```python
from build123d import *

# Parameters (mm, degrees)
F0_R     = 44.45
F1_DEPTH = 9.525
F2_R     = 2.0828
F3_DEPTH = 25.4
F4_R     = 3.6322
F5_DEPTH = 4.1656
F6_R     = 2.38125
F7_R     = 12.7


with BuildPart() as f1:
    # F0 (on Top) → F1 (new body)
    with BuildSketch(Plane.XY):
        with BuildLine():
            Line((-25.4, 90.4875), (-25.4, 43.994091))
            ThreePointArc((-25.4, 43.994091), (0, -50.8), (25.4, 43.994091))
            Line((25.4, 43.994091), (25.4, 90.4875))
            Line((25.4, 90.4875), (-25.4, 90.4875))
        make_face()
        Circle(F0_R, mode=Mode.SUBTRACT)
    extrude(amount=F1_DEPTH)

    # F2 (on face) → F3 (cut)
    with BuildSketch(Plane.XY.offset(9.525)):
        with Locations((-20.6375, 84.1375)):
            Circle(F2_R)
        with Locations((20.6375, 84.1375)):
            Circle(F2_R)
        with Locations((20.6375, 53.9623)):
            Circle(F2_R)
        with Locations((-20.6375, 53.9623)):
            Circle(F2_R)
    extrude(amount=-F3_DEPTH, mode=Mode.SUBTRACT)

    # F4 (on face) → F5 (cut)
    with BuildSketch(Plane.XY.offset(9.525)):
        with Locations((-20.6375, 84.1375)):
            Circle(F4_R)
        with Locations((20.6375, 84.1375)):
            Circle(F4_R)
        with Locations((20.6375, 53.9623)):
            Circle(F4_R)
        with Locations((-20.6375, 53.9623)):
            Circle(F4_R)
    extrude(amount=-F5_DEPTH, mode=Mode.SUBTRACT)

    # F6
    f6_edges = [f1.edges().sort_by_distance(p)[0] for p in [
        (-25.4, 90.4875, 4.7625),
        (25.4, 90.4875, 4.7625),
    ]]
    fillet(f6_edges, radius=F6_R)

    # F7
    f7_edges = [f1.edges().sort_by_distance(p)[0] for p in [
        (-25.4, 43.994091, 4.7625),
        (25.4, 43.994091, 4.7625),
    ]]
    fillet(f7_edges, radius=F7_R)


solid = f1.part
```
Design review of the part built by this model. Coordinates are the model's own, in mm. A direction names the side the tool comes from. Coordinates: 2 decimals unless noted, no trailing zeros. Loops run counter-clockwise (first coordinate to the right, second up) from the corner with the lowest first, then second, coordinate; pieces in that order, holes last.
Q1. We need section C-C on z = 1.5. State the section outline as (x, y) points, and give its area (3 significant figures).
Reported:
outline: (-30.48, 40.64) arc R50.8 ccw (long way) to (30.48, 40.64) arc R12.7 cw to (25.4, 50.8) - (25.4, 88.11) arc R2.38 ccw to (23.02, 90.49) - (-23.02, 90.49) arc R2.38 ccw to (-25.4, 88.11) - (-25.4, 50.8) arc R12.7 cw to start; hole circle Ø88.9 at (0, 0); hole circle Ø4.17 at (-20.64, 53.96); hole circle Ø4.17 at (-20.64, 84.14); hole circle Ø4.17 at (20.64, 53.96); hole circle Ø4.17 at (20.64, 84.14)
area: 3,980 mm2
Q2. Tool access review of faces 4 (the face through (25.4, 69, 5)), 5 (the face through (19.85, 50.416, 7.471)), 6 (the face through (-21.09, 51.93, 2.72)), 7 (the face through (-25.4, 70, 5)), 8 (the face through (0, 46, 9.525)): name each direction out of +Z, -Z, +X, -X, +Y, -Y from which nothing blocks a thin tool from reaching the whole face with its end or side.
Reported:
face 4: +Z, -Z, +X, +Y
face 5: +Z
face 6: +Z, -Z
face 7: +Z, -Z, -X, +Y
face 8: +Z, +X, -X, +Y, -Y
Q3. For pin 1 (4 mm diameter, centred on y = -14.5, z = 4, fed in from -X); pin 2 (3.5 mm diameter, centred on x = 20.64, y = 53.96, fed in from +Z); pin 3 (6.5 mm diameter, centred on x = 20.64, y = 84.14, fed in from +Z); pin 4 (2 mm diameter, centred on x = 14, z = 8, fed in from -Y), all flat-tipped, find the tip position at first contact; note any pin that passes through.
Reported:
pin 1: stops at x = -49.24
pin 2: passes through
pin 3: stops at z = 5.36
pin 4: stops at y = -49.11
Q4. To check wall thickness, follow line 1 (X direction, y = 51, z = 7.25); line 2 (Y direction, x = 20.5, z = 1.75); line 3 (X direction, y = 61, z = 3.5). State the ranges of each line that lie inside material, in increasing order.
Reported:
line 1: x = -25.4 to -22.74, -18.54 to 18.54, 22.74 to 25.4
line 2: y = -46.48 to -39.44, 39.44 to 51.88, 56.04 to 82.06, 86.22 to 90.49
line 3: x = -25.4 to 25.4
Q5. We need section B-B on y = 0. State the section outline as (x, z) points (3 decimals).
Reported:
outline: (-50.8, 0) - (-44.45, 0) - (-44.45, 9.525) - (-50.8, 9.525) - close; (44.45, 0) - (50.8, 0) - (50.8, 9.525) - (44.45, 9.525) - close
Q6. The part is to be moulded in two halves that separate along X. For faces 1 (the face through (20.2, 82.1, 2.7)), 2 (the face through (-26.7, 45.2, 4.8)), 3 (the face through (-1.78, -50.77, 4.7)), say which applies: +X half, -X half, draft (parallel to the pull), parting line (faces both ways), or undercut.
Reported:
face 1: undercut
face 2: -X half
face 3: parting line
